Answer from the drawing. Dimensions are ordinates in mm from the lowest x, y and z of the part. Give positions to 0.01 mm unless a question says otherwise; leave off trailing zeros. Loops run counter-clockwise (first coordinate to the right, second up) from the corner with the lowest first, then second, coordinate; pieces in that order, holes last. Notation, with made-up numbers: M 82,-31.75 L 97,-31.75 A23 cw 97,-8.75 Z; hole C 65,15 d9. An arc over 180 degrees is marked long. Use a Markdown table: item, result.
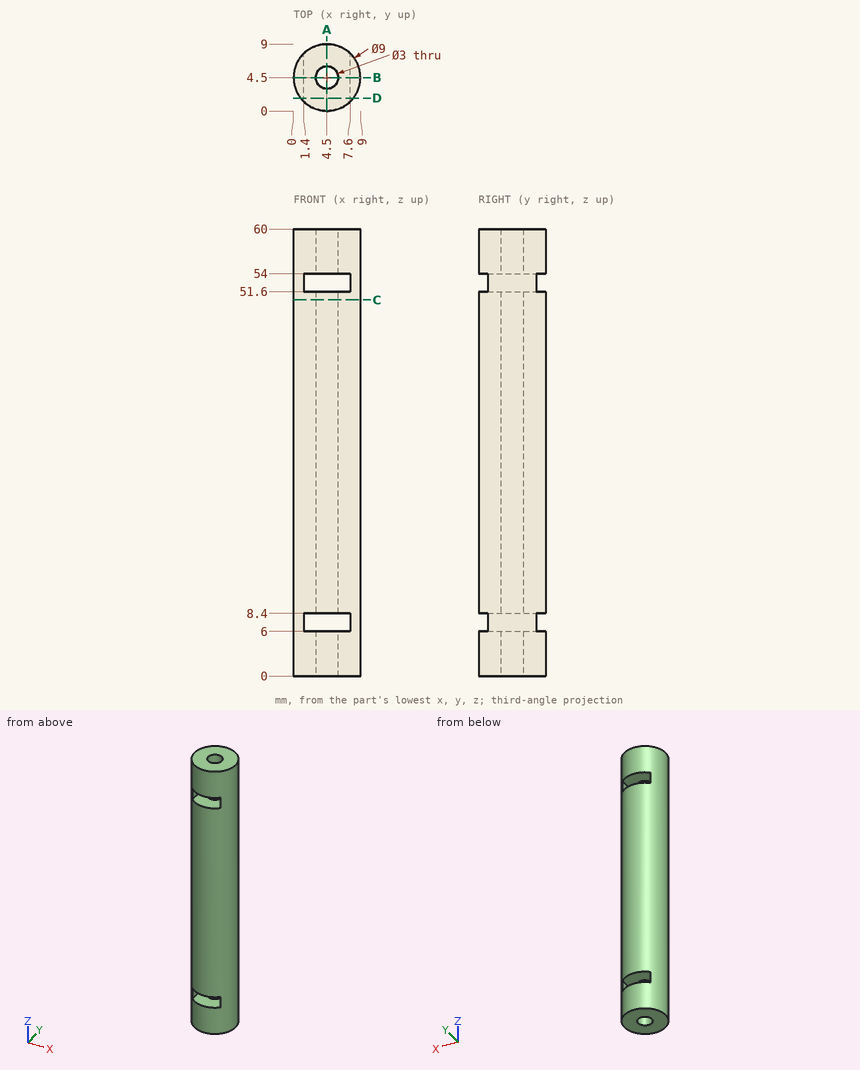
(1) Given P1, Ø1, axis at x = 3.5, z = 25.5, coming from the +Y side; P2, Ø1.2, axis at y = 3.5, z = 6.5, coming from the +X side; P3, Ø3, axis at x = 8, z = 20.5, coming from the -Y side, each flat-ended and moving along its own axis, determine where each tip first touches the part or whether it passes through.
Entries:
| item | result |
|---|---|
| P1 | stops at y = 8.97 |
| P2 | stops at x = 8.98 |
| P3 | stops at y = 0.47 |
(2) A cutting plane is placed at C-C (z = 50.5). Write down the section's boundary in (x, y).
Entries:
| item | result |
|---|---|
| outline | C 4.5,4.5 d9; hole C 4.5,4.5 d3 |
(3) Consider probe 1 along Z at (x, y) = (5.25, 8.5); probe 2 along Y at (x, z) = (4.5, 25.5); probe 3 along X at (y, z) = (4.25, 37.5). Determine where each line is inside the solid, lowest interval first. Write a range as [from, to].
Entries:
| item | result |
|---|---|
| probe 1 | z = [0, 6], [8.4, 51.6], [54, 60] |
| probe 2 | y = [0, 3], [6, 9] |
| probe 3 | x = [0.01, 3.02], [5.98, 8.99] |
(4) A cutting plane is placed at D-D (y = 1.75). Write down the section's boundary in (x, z), and give its area (3 significant figures).
Entries:
| item | result |
|---|---|
| outline | M 0.94,0 L 8.06,0 L 8.06,60 L 0.94,60 Z; hole M 1.4,6 L 7.6,6 L 7.6,8.4 L 1.4,8.4 Z; hole M 1.4,51.6 L 7.6,51.6 L 7.6,54 L 1.4,54 Z |
| area | 398 mm² |
(5) A cutting plane is placed at A-A (x = 4.5). Write down the section's boundary in (y, z), and give its area (3 significant figures).
Entries:
| item | result |
|---|---|
| outline | M 0,0 L 3,0 L 3,6 L 0,6 Z; M 0,8.4 L 3,8.4 L 3,51.6 L 0,51.6 Z; M 0,54 L 3,54 L 3,60 L 0,60 Z; M 6,0 L 9,0 L 9,6 L 6,6 Z; M 6,8.4 L 9,8.4 L 9,51.6 L 6,51.6 Z; M 6,54 L 9,54 L 9,60 L 6,60 Z |
| area | 331 mm² |
(6) A cutting plane is placed at B-B (y = 4.5). Write down the section's boundary in (x, z).
Entries:
| item | result |
|---|---|
| outline | M 0,0 L 3,0 L 3,6 L 1.4,6 L 1.4,8.4 L 3,8.4 L 3,51.6 L 1.4,51.6 L 1.4,54 L 3,54 L 3,60 L 0,60 Z; M 6,0 L 9,0 L 9,60 L 6,60 L 6,54 L 7.6,54 L 7.6,51.6 L 6,51.6 L 6,8.4 L 7.6,8.4 L 7.6,6 L 6,6 Z |
